CAD build for the part. Positions are in the model's coordinates, mm. A direction names the side the tool comes from. Coordinates: 2 decimals unless noted, no trailing zeros. Loops run counter-clockwise (first coordinate to the right, second up) from the corner with the lowest first, then second, coordinate; pieces in that order, holes last. Notation, with made-up numbers: (-1.5, 3) -> (25.5, 3) arc R25 ccw to (25.5, 19) -> close; hole circle Ø3 at (79, -19). An arc over 180 degrees is marked (long way). Write item = value, one per line. Start each with the question number.
(1) Tool access for faces 5 (the face through (-0.1, -16.5, 1.588)), 6 (the face through (-13.81, 14.81, -3.2)), 7 (the face through (-14.857, 0.157, -5.897)), 8 (the face through (13.89, 14.73, -3.2)), 9 (the face through (12.751, -13.623, -3.219)): list every direction of +Z, -Z, +X, -X, +Y, -Y with a clear straight run to the whole face (end or side of a thin tool).
(2) Drill centre lines: line 1 (Y direction, x = 0, z = 5.35); line 2 (X direction, y = 3, z = -1.5); line 3 (Y direction, x = -3.5, z = -4.5). Where is each one in solid material? Low to high. Write a range as from..to.
(3) Band-saw the part on D-D (z = 4). Write the cut outline in (x, y).
(4) Flat gauge pins, fed straight in: P1, Ø1.9, axis at x = 5, z = -2, coming from the +Y side; P2, Ø3, axis at y = -1.5, z = -2, coming from the -X side; P3, Ø2.5, axis at y = 4, z = -4, coming from the +X side. Where does each tip first touch, or does it go through?
(5) Pull direction Y, two halves, no side cores. Call faces 1 (the face through (0, 14.674, -3)), 2 (the face through (-0.14, -15.78, -5.9)), 3 (the face through (-15.334, 0, -3)), 4 (the face through (0, -14.674, -3)): +Y half, -Y half, draft (parallel to the pull), parting line (faces both ways), or undercut.
(6) Band-saw the part on C-C (z = -3.75). Write the cut outline in (x, y) (1 decimal), and give its area (3 significant figures).
```python
from build123d import *

# Parameters (mm, degrees)
F0_R     = 27.4307553129
F1_DEPTH = 6.35
F9_R     = 5.08
F2_T     = -1.5875
F3_W     = 30.6679024691
F3_H     = 32.5223739966
F4_DEPTH = 6.35
F5_R     = 5.08
F6_T     = -1.5875
F7_DEPTH = 6.351
F10_R    = 1.5875
F11_R    = 1.58749


# Not quite as in the source:
# - a fillet or chamfer is up to 0.001 mm smaller than in the source, because OpenCascade refuses the exact size


with BuildPart() as f1:
    # F0 (on Top) → F1 (new body)
    with BuildSketch(Plane.XY):
        Circle(F0_R)
    extrude(amount=F1_DEPTH)

    # F9
    f9_edges = [f1.edges().sort_by_distance(p)[0] for p in [
        (-27.430755, 0, 0),
    ]]
    fillet(f9_edges, radius=F9_R)

    # F2
    f2_openings = [f1.faces().sort_by_distance(p)[0] for p in [
        (0, 0, 6.35),
    ]]
    offset(amount=F2_T, openings=f2_openings)

    # F3 (on face) → F4 (join)
    with BuildSketch(Plane(origin=(0, 0, 0), x_dir=(1, 0, 0), z_dir=(0, 0, -1))):
        Rectangle(F3_W, F3_H)
    extrude(amount=F4_DEPTH)

    # F5
    f5_edges = [f1.edges().sort_by_distance(p)[0] for p in [
        (-15.333951, 16.261187, -3.175),
        (-15.333951, -16.261187, -3.175),
        (15.333951, -16.261187, -3.175),
        (15.333951, 16.261187, -3.175),
    ]]
    fillet(f5_edges, radius=F5_R)

    # F6
    f6_openings = [f1.faces().sort_by_distance(p)[0] for p in [
        (0, 0, -6.35),
    ]]
    offset(amount=F6_T, openings=f6_openings, kind=Kind.INTERSECTION)

    # F7 (cut, through all): a face of the model
    f7_faces = [f1.faces().sort_by_distance(p)[0] for p in [
        (0, 0, 0),
    ]]
    extrude(f7_faces, amount=-F7_DEPTH, mode=Mode.SUBTRACT)

    # F10
    f10_edges = [f1.edges().sort_by_distance(p)[0] for p in [
        (13.746451, 0, 1.5875),
    ]]
    fillet(f10_edges, radius=F10_R)

    # F11 (radius 1.5875 in the source; OpenCascade refuses exactly that, so slightly less here)
    f11_edges = [f1.edges().sort_by_distance(p)[0] for p in [
        (15.333951, 0, 0),
        (15.333951, 11.181187, -3.175),
        (15.333951, -11.181187, -3.175),
        (15.333951, 0, -6.35),
    ]]
    fillet(f11_edges, radius=F11_R)


solid = f1.part
```
Findings below:
q1.face_5 = +Z
q1.face_6 = -Z, -X, +Y
q1.face_7 = -Z, -X, +Y, -Y
q1.face_8 = -Z, +X, +Y
q1.face_9 = +Z, -Z
q2.line_1 = -27.43..-25.84, 25.84..27.43
q2.line_2 = -15.34..-13.75, 13.75..15.34
q2.line_3 = -16.26..-14.67, 14.67..16.26
q3.outline = circle Ø54.63 at (0, 0); hole circle Ø51.34 at (0, 0)
q4.P1 = 16.35
q4.P2 = -15.76
q4.P3 = 15.33
q5.face_1 = undercut
q5.face_2 = -Y half
q5.face_3 = draft
q5.face_4 = undercut
q6.outline = (-15.3, -11.2) arc R5.1 ccw to (-10.3, -16.3) -> (10.3, -16.3) arc R5.1 ccw to (15.3, -11.2) -> (15.3, 11.2) arc R5.1 ccw to (10.3, 16.3) -> (-10.3, 16.3) arc R5.1 ccw to (-15.3, 11.2) -> close; hole (-13.7, -11.2) arc R3.5 ccw to (-10.3, -14.7) -> (10.3, -14.7) arc R3.5 ccw to (13.7, -11.2) -> (13.7, 11.2) arc R3.5 ccw to (10.3, 14.7) -> (-10.3, 14.7) arc R3.5 ccw to (-13.7, 11.2) -> close
q6.area = 179 mm²
